Work out the finished part from the listing and answer in its coordinate system (mm). Coordinates: 2 decimals unless noted, no trailing zeros. Loops run counter-clockwise (first coordinate to the right, second up) from the corner with the lowest first, then second, coordinate; pieces in that order, holes last. Notation, with made-up numbers: (-12.75, 67) - (41.25, 67) arc R17 cw to (41.25, 86) - close; hole circle Ø4 at (-3, 59.25). An arc over 180 degrees is marked (long way). Write each question's results on one line, items separated by ' | '. Start each with the question number.
1. A cutting plane is placed at C-C on z = 2.35. Determine the outline of the cut face in (x, y) (3 decimals).
2. Find the intervals of material crossed by line 1 along Y through (x, z) = (0, 1.1); line 2 along X through (y, z) = (-1, 2.7); line 3 along X through (y, z) = (-16, 2.1), in increasing order. Write a range as [from, to].
3. A cutting plane is placed at A-A on y = 0. Determine the outline of the cut face in (x, z) (3 decimals).
4. Each of these flat-tipped pins is pushed along its axis until it touches: P1, Ø2, axis at x = 7, y = 25.5, coming from the -Z side; P2, Ø3, axis at x = -28.575, y = 0, coming from the +Z side; P3, Ø1.5, axis at y = 26, z = 1, coming from the +X side. Where does it stop, or does it pass through?
5. A cutting plane is placed at D-D on y = -12. Determine the outline of the cut face in (x, z) (3 decimals), then the cut area to 3 significant figures.
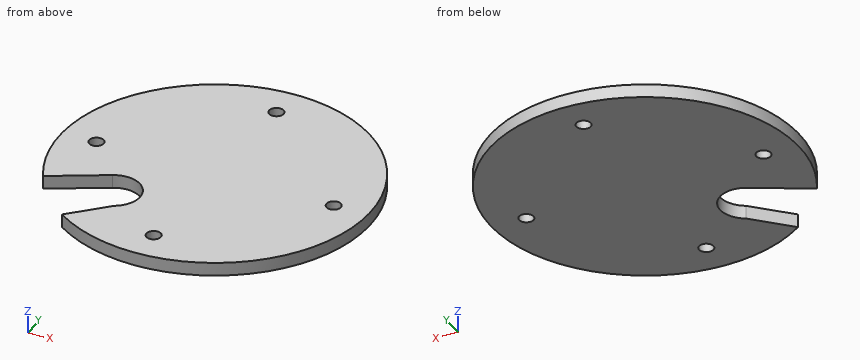
from build123d import *

# Parameters (mm, degrees)
F0_R     = 36.83
F1_DEPTH = 3.175
F3_D     = 3.4544
F3_DEPTH = 11.43
F3_TIP   = 1.0378064612
F4_R     = 6.35
F5_DEPTH = 3.176
F7_DEPTH = 3.176


with BuildPart() as f1:
    # F0 (on Top) → F1 (new body)
    with BuildSketch(Plane.XY):
        Circle(F0_R)
    extrude(amount=F1_DEPTH)

    # F3
    with Locations(Plane.XY.offset(3.175)):
        with Locations((-28.575, 0), (0, 28.575), (28.575, 0), (0, -28.575)):
            Hole(F3_D / 2, depth=F3_DEPTH)
            with Locations((0, 0, -(F3_DEPTH + F3_TIP / 2))):  # 118° drill point
                Cone(0, F3_D / 2, F3_TIP, mode=Mode.SUBTRACT)

    # F4 (on face) → F5 (cut, through all)
    with BuildSketch(Plane.XY.offset(3.175)):
        with Locations((-16.1644610179, -16.1644610179)):
            Circle(F4_R)
    extrude(amount=-F5_DEPTH, mode=Mode.SUBTRACT)

    # F6 (on face) → F7 (cut, through all)
    with BuildSketch(Plane.XY.offset(3.175)):
        Polygon((-10.6037825397, -19.2306239069), (-19.2306239069, -10.6037825397), (-32.2519351736, -17.7837447563), (-39.33729292, -25.7967901035), (-21.3696253197, -29.9964666869), align=None)
    extrude(amount=-F7_DEPTH, mode=Mode.SUBTRACT)


solid = f1.part
Values:
1) outline: (-32.252, -17.784) - (-19.231, -10.604) arc R6.35 cw to (-13.098, -21.725) - (-21.37, -29.996) arc R36.83 ccw (long way) to start; hole circle Ø3.454 at (-28.575, 0); hole circle Ø3.454 at (0, -28.575); hole circle Ø3.454 at (0, 28.575); hole circle Ø3.454 at (28.575, 0)
2) line 1: [-36.83, -30.3], [-26.85, 26.85], [30.3, 36.83] | line 2: [-36.82, -29.98], [-27.17, 27.17], [29.98, 36.82] | line 3: [-33.17, -29.02], [-9.82, 33.17]
3) outline: (-36.83, 0) - (-30.302, 0) - (-30.302, 3.175) - (-36.83, 3.175) - close; (-26.848, 0) - (26.848, 0) - (26.848, 3.175) - (-26.848, 3.175) - close; (30.302, 0) - (36.83, 0) - (36.83, 3.175) - (30.302, 3.175) - close
4) P1: z = 0 | P2: through | P3: x = 26.81
5) outline: (-34.82, 0) - (-21.763, 0) - (-21.763, 3.175) - (-34.82, 3.175) - close; (-11.371, 0) - (34.82, 0) - (34.82, 3.175) - (-11.371, 3.175) - close | area: 188 mm^2
